Check sheet for the modelled part. Datum: model origin and axes. Units: mm. A direction names the side the tool comes from. Give positions to 0.01 mm unless a question says otherwise; leave off trailing zeros. Order: outer loops, then holes, each group sorted by start corner. A loop starts at its lowest first (then second) coordinate and runs counter-clockwise, first axis right, second up. Notation, with made-up numbers: (-8, -12.75) -> (10, -12.75) arc R28 cw to (10, 5.25) -> close; hole circle Ø2 at (2, 52). An arc over 180 degrees is marked (long way). Answer in a Markdown table with one row per item. Add a question column.
(1) Cross-section at D-D (y = 82). Record the cut outline in (x, z).
(2) Cross-section at C-C (z = 12). Record the cut outline in (x, y).
(3) Thickness scan on L1, parallel to X at y = 10.5, z = 67; L2, parallel to Y at x = 37.5, z = 4; L3, parallel to X at y = 66.5, z = -44. Record the ranges inside material, lowest first. Write a range as [from, to].
(4) Cross-section at A-A (y = -55.5). Record the cut outline in (x, z).
(5) Set-up check for faces 1 (the face through (154.618, -1, 1)), 2 (the face through (107.996, -92.877, 1.024)): record each of +Z, -Z, +X, -X, +Y, -Y from which the full face is reachable in a straight line by a thin tool's end or side.
(6) Release check for a two-part mould opening along Y. For faces 3 (the face through (20, -9, -73.15)), 4 (the face through (109.09, 92.14, 1.02)), 5 (the face through (113.69, 97.485, 1.024)) record: released by +Y, released by -Y, zero draft, split by the parting line, or undercut.
(7) Go/stop test with flat-tipped pins: pin 1 (4 mm diameter, centred on x = 77.5, z = -34.5, fed in from +Y); pin 2 (12 mm diameter, centred on x = 133.5, z = 47.5, fed in from -Y); pin 3 (12 mm diameter, centred on x = 87.5, z = -52, fed in from -Y). Record where each tip stops, or that it passes through.
(8) Cross-section at B-B (x = 56). Record the cut outline in (y, z).
```python
from build123d import *

# Parameters (mm, degrees)
SALIENTE_EXTRUIR1_DEPTH = 73.15


with BuildPart() as part:
    # Croquis1 → Saliente-Extruir1 (new body, symmetric)
    with BuildSketch(Plane.XY):
        Polygon((154.617693897, 70), (71.6, 125.75), (0, 125.75), (0, 76.55), (16, 95.55), (16, -95.55), (0, -76.55), (0, -125.75), (71.6, -125.75), (154.617693897, -70), align=None)
        Polygon((147.617693897, 66.26886769), (69.467692507, 118.75), (23, 118.75), (23, -118.75), (69.467692507, -118.75), (147.617693897, -66.26886769), align=None, mode=Mode.SUBTRACT)
    extrude(amount=SALIENTE_EXTRUIR1_DEPTH, both=True)


solid = part.part
```
Answer below:
| question | item | result |
|---|---|---|
| 1 | outline | (0, -73.15) -> (4.59, -73.15) -> (4.59, 73.15) -> (0, 73.15) -> close; (16, -73.15) -> (23, -73.15) -> (23, 73.15) -> (16, 73.15) -> close; (124.19, -73.15) -> (136.75, -73.15) -> (136.75, 73.15) -> (124.19, 73.15) -> close |
| 2 | outline | (0, -125.75) -> (71.6, -125.75) -> (154.62, -70) -> (154.62, 70) -> (71.6, 125.75) -> (0, 125.75) -> (0, 76.55) -> (16, 95.55) -> (16, -95.55) -> (0, -76.55) -> close; hole (23, -118.75) -> (69.47, -118.75) -> (147.62, -66.27) -> (147.62, 66.27) -> (69.47, 118.75) -> (23, 118.75) -> close |
| 3 | L1 | x = [16, 23], [147.62, 154.62] |
| 3 | L2 | y = [-125.75, -118.75], [118.75, 125.75] |
| 3 | L3 | x = [16, 23], [147.27, 154.62] |
| 4 | outline | (16, -73.15) -> (23, -73.15) -> (23, 73.15) -> (16, 73.15) -> close; (147.62, -73.15) -> (154.62, -73.15) -> (154.62, 73.15) -> (147.62, 73.15) -> close |
| 5 | face 1 | +Z, -Z, +X, +Y, -Y |
| 5 | face 2 | +Z, -Z |
| 6 | face 3 | zero draft |
| 6 | face 4 | undercut |
| 6 | face 5 | released by +Y |
| 7 | pin 1 | stops at y = 123.13 |
| 7 | pin 2 | stops at y = -88.21 |
| 7 | pin 3 | stops at y = -119.1 |
| 8 | outline | (-125.75, -73.15) -> (-118.75, -73.15) -> (-118.75, 73.15) -> (-125.75, 73.15) -> close; (118.75, -73.15) -> (125.75, -73.15) -> (125.75, 73.15) -> (118.75, 73.15) -> close |
